Read the model definition and answer for the solid it produces. Units are mm, in the model's axes. A direction names the side the tool comes from. Coordinates: 2 decimals unless noted, no trailing zeros. Order: outer loops, then holes, each group sorted by start corner. A loop starts at its lowest first (then second) coordinate and runs counter-clockwise, first axis right, second up.
Autodesk Inventor part; units mm, degrees
ref_plane "YZ Plane" through (0, 0, 0) normal (1, 0, 0) x (0, 1, 0)
ref_plane "XZ Plane" through (0, 0, 0) normal (0, 1, 0) x (-1, 0, 0)
ref_plane "XY Plane" through (0, 0, 0) normal (0, 0, 1) x (1, 0, 0)
sketch "スケッチ9" plane through (0, 0, 0) normal (0, 1, 0) x (-1, 0, 0)
  line L0 (5, 7.5) -> (-5, 7.5)
  line L1 (-5, 7.5) -> (-5, -7.5)
  line L2 (-5, -7.5) -> (5, -7.5)
  line L3 (5, -7.5) -> (5, 7.5)
  line L4 (7, 0) -> (-7, 0)
  line L5 (0, -10.5) -> (0, 10.5)
  point P0 (0, 0)
  point P1 (5, 0)
  point P2 (0, 7.5)
  dimension "d53" = 15
  dimension "d54" = 10
extrude "プレート7" add sketch "スケッチ9" along normal blind 1
sketch "スケッチ10" plane through (-5, 0, -6.5) normal (0, 0, -1) x (-1, 0, 0)
  line L0 (-10, 0) -> (0, 0)
  line L1 (0, 0) -> (0, 15)
  line L2 (0, 15) -> (-10, 15)
  line L3 (-10, 15) -> (-10, 0)
edge flange "フランジ5" height 15 angle 90 thickness 1 bend radius 1 thickness toward (0, 0, -1) relief tear relief width 1 relief depth 0.5 edges at (0, 1, -7.5) wall of the first edge with corners at (5, 0, -6.5) (-5, 0, -6.5) (-5, 15, -6.5) (5, 15, -6.5)
bend "曲げ5"
corner "コーナー5"
sketch "スケッチ11" plane through (-5, 15, -6.5) normal (0, 0, 1) x (1, 0, 0)
  circle A0 centre (5, -6) radius 2.5
  line L0 (10, 0) -> (0, 0)
  line L1 (0, 0) -> (0, -13)
  point P0 (5, -15)
  dimension "d66" = 5
  dimension "d67" = 6
  dimension "d76" = 5
sketch "スケッチ12" plane through (0, 1, 0) normal (0, 1, 0) x (1, 0, 0)
  circle A0 centre (0, -1.5) radius 2.5
  line L0 (5, -7.5) -> (-5, -7.5)
  line L1 (-5, -7.5) -> (-5, 5.5)
  line L2 (0, 11.6) -> (0, -13.6)
  point P0 (0, 0)
  dimension "d69" = 6
  dimension "d71" = 5
extrude "押し出し3" cut sketch "スケッチ12" against normal up to next
extrude "押し出し4" cut sketch "スケッチ11" against normal up to next
fillet "フィレット2" radius 2 2 edges at (5, 0.5, 7.5) (-5, 0.5, 7.5)
equation "\"d55\" = Thickness"
equation "\"d56\" = BendReliefWidth"
equation "\"d57\" = BendReliefDepth"
equation "\"d58\" = MinimumRemnant"
equation "\"d59\" = TransitionRadius"
equation "\"d62\" = BendRadius"
equation "\"d63\" = CornerReliefSize"
equation "\"d64\" = GapSize"
equation "\"d65\" = JacobiRadiusSize"
equation "\"BendRadius\" = Thickness"
equation "\"BendReliefWidth\" = Thickness"
equation "\"BendReliefDepth\" = 0.5 * Thickness"
equation "\"CornerReliefSize\" = 4 * Thickness"
equation "\"MinimumRemnant\" = 2 * Thickness"
equation "\"TransitionRadius\" = BendRadius"
equation "\"JacobiRadiusSize\" = BendRadius"
equation "\"GapSize\" = Thickness"
properties part number "element_clip" material "アルミニウム 6061"
1) Straight lines are drawn through the part: line 1 (Z direction, x = 2.75, y = 2.25); line 2 (Y direction, x = -0.5, z = 5.5); line 3 (X direction, y = 0.55, z = 1.5). For each, find the intervals that lie inside material, in ascending order.
A:
line 1: z = -7.5 to -6.5
line 2: y = 0 to 1
line 3: x = -5 to -2.5, 2.5 to 5
2) A cutting plane is placed at C-C, the plane x = 2. Determine the outline of the cut face in (y, z), and give its area (3 significant figures).
A:
outline: (0, -5.5) arc R2 ccw to (2, -7.5) - (7.5, -7.5) - (7.5, -6.5) - (2, -6.5) arc R1 cw to (1, -5.5) - (1, 0) - (0, 0) - close; (0, 3) - (1, 3) - (1, 7.5) - (0, 7.5) - close; (10.5, -7.5) - (15, -7.5) - (15, -6.5) - (10.5, -6.5) - close
area: 22.4 mm2
3) A cutting plane is placed at A-A, the plane z = 1.5. Determine the outline of the cut face in (x, y).
A:
outline: (-5, 0) - (-2.5, 0) - (-2.5, 1) - (-5, 1) - close; (2.5, 0) - (5, 0) - (5, 1) - (2.5, 1) - close
4) Flat-ended cylindrical pins translate along their axes: pin 1 Ø6 at (x, z) = (0, 1.5) entering from +Y; pin 2 Ø6 at (x, y) = (0, 9) entering from +Z. Find the tip coordinate at first contact, or state that the pin passes through.
A:
pin 1: stops at y = 1
pin 2: stops at z = -6.5
5) Which of the six approach directions +Z, -Z, +X, -X, +Y, -Y give full straight-line access (tool end or side, diameter ignored) to faces 1 (the flat face through (5, 4, -7)), 2 (the flat face through (-2.2, 1, -0.4))?
A:
face 1: +Z, -Z, +X, +Y, -Y
face 2: +Z, +X, -X, +Y
6) Determine the mould class of faces 3 (the cylindrical face through (-0.54, 6.56, -6.99)), 4 (the cylindrical face through (-0.07, 0.6, -6.93)), 5 (the cylindrical face through (-0.07, 1.301, -6.215)), 6 (the flat face through (-5, 4, -7)) for opening direction Y: pulls with the +Y half, pulls with the -Y half, needs draft (parallel to the pull), parting line crosses it, or undercut.
A:
face 3: undercut
face 4: pulls with the -Y half
face 5: pulls with the +Y half
face 6: needs draft
7) A cutting plane is placed at B-B, the plane y = 9. Determine the outline of the cut face in (x, z).
A:
outline: (-5, -7.5) - (-2.5, -7.5) - (-2.5, -6.5) - (-5, -6.5) - close; (2.5, -7.5) - (5, -7.5) - (5, -6.5) - (2.5, -6.5) - close
8) A cutting plane is placed at D-D, the plane x = -2.75. Determine the outline of the cut face in (y, z), and give its area (3 significant figures).
A:
outline: (0, -5.5) arc R2 ccw to (2, -7.5) - (15, -7.5) - (15, -6.5) - (2, -6.5) arc R1 cw to (1, -5.5) - (1, 7.5) - (0, 7.5) - close
area: 28.4 mm2
